```python
from build123d import *

# Parameters (mm, degrees)
BOSS_EXTRUDE1_DEPTH          = 1305
FILLET1_R                    = 7
F_7_0_7_DIAMETER_HOLE1_D     = 7
F_7_0_7_DIAMETER_HOLE1_DEPTH = 6.3
LPATTERN1_COUNT              = 3
LPATTERN1_PITCH              = 32.5
LPATTERN1_COUNT_DIR2         = 2
LPATTERN1_PITCH_DIR2         = 52


with BuildPart() as part:
    # Sketch1 → Boss-Extrude1 (new body, symmetric)
    with BuildSketch(Plane.XY):
        Polygon((0, 60), (0, -60), (-32, -60), (-32, -53.7), (-2.2, -53.7), (-2.2, 53.7), (-32, 53.7), (-32, 60), align=None)
    boss_extrude1 = extrude(amount=BOSS_EXTRUDE1_DEPTH, both=True)

    # Mirror1: Boss-Extrude1 across plane
    add(boss_extrude1.mirror(Plane(origin=(0, 60, 1305), x_dir=(0, 0, 1), z_dir=(-1, 0, 0))))

    # Fillet1
    fillet1_edges = [part.edges().sort_by_distance(p)[0] for p in [
        (-2.2, -53.7, 0),
        (-2.2, 53.7, 0),
        (2.2, -53.7, 0),
        (2.2, 53.7, 0),
    ]]
    fillet(fillet1_edges, radius=FILLET1_R)

    # Ø7.0 (7) Diameter Hole1
    with Locations(Plane(origin=(0, -60, 0), x_dir=(-1, 0, 0), z_dir=(0, -1, 0))):
        with Locations((-26, -1132.5)):
            f_7_0_7_diameter_hole1 = Hole(F_7_0_7_DIAMETER_HOLE1_D / 2, depth=F_7_0_7_DIAMETER_HOLE1_DEPTH)

    # LPattern1: 7.0 _7_ Diameter Hole1 3 × 2
    with Locations(*[(-j * LPATTERN1_PITCH_DIR2, 0, -i * LPATTERN1_PITCH) for i in range(LPATTERN1_COUNT) for j in range(LPATTERN1_COUNT_DIR2) if (i, j) != (0, 0)]):
        add(f_7_0_7_diameter_hole1, mode=Mode.SUBTRACT)


solid = part.part
```
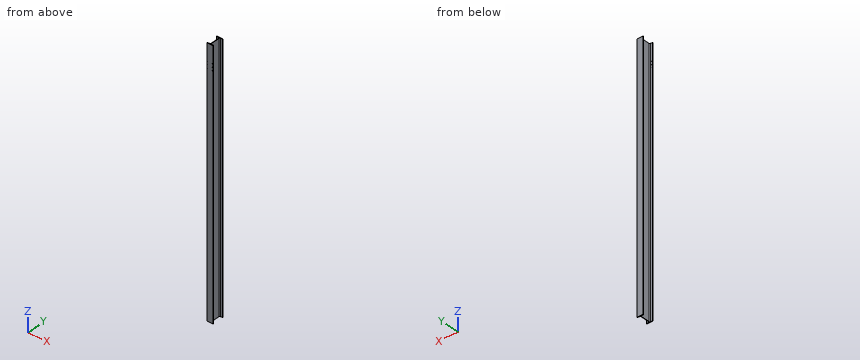
Geometry check sheet. Reference: the model listing, model coordinates, mm. Give positions to 0.01 mm unless a question says otherwise; leave off trailing zeros. Order: outer loops, then holes, each group sorted by start corner. A loop starts at its lowest first (then second) coordinate and runs counter-clockwise, first axis right, second up. Notation, with made-up numbers: (89, 76.5) - (120, 76.5) arc R21 cw to (120, 95.5) - close; hole circle Ø7 at (-14.75, -8). An arc over 180 degrees is marked (long way). Answer in a Markdown table with one row per item. Add a question column.
Q1. Material ranges on probe 1 along X at (y, z) = (-55.5, 1067.5); probe 2 along Z at (x, y) = (26, -55.25); probe 3 along Y at (x, z) = (8, 620), recorded low to high. Write a range as from..to.
Q2. Gauge pin test, flat ends, axial feed: pin 1 (6 mm diameter, centred on y = -20.5, z = 160, fed in from +X); pin 2 (2 mm diameter, centred on y = 43.5, z = -614.5, fed in from -X); pin 3 (5.5 mm diameter, centred on x = 26, z = 1067.5, fed in from -Y). Record the tip position at first contact, or that the pin passes through.
Q3. Cross-section at A-A, the plane z = 551. Enter the section's corners in (x, y).
Q4. Cross-section at B-B, the plane y = 17. Enter the section's corners in (x, z), then the cut area to 3 significant figures.
Check values:
| question | item | result |
|---|---|---|
| 1 | probe 1 | x = -32..-29.5, -22.5..22.5, 29.5..32 |
| 1 | probe 2 | z = -1305..1064, 1071..1096.5, 1103.5..1129, 1136..1305 |
| 1 | probe 3 | y = -60..-53.6, 53.6..60 |
| 2 | pin 1 | stops at x = 2.2 |
| 2 | pin 2 | stops at x = -2.2 |
| 2 | pin 3 | stops at y = 53.7 |
| 3 | outline | (-32, -60) - (32, -60) - (32, -53.7) - (9.2, -53.7) arc R7 cw to (2.2, -46.7) - (2.2, 46.7) arc R7 cw to (9.2, 53.7) - (32, 53.7) - (32, 60) - (-32, 60) - (-32, 53.7) - (-9.2, 53.7) arc R7 cw to (-2.2, 46.7) - (-2.2, -46.7) arc R7 cw to (-9.2, -53.7) - (-32, -53.7) - close |
| 4 | outline | (-2.2, -1305) - (2.2, -1305) - (2.2, 1305) - (-2.2, 1305) - close |
| 4 | area | 11,500 mm^2 |
